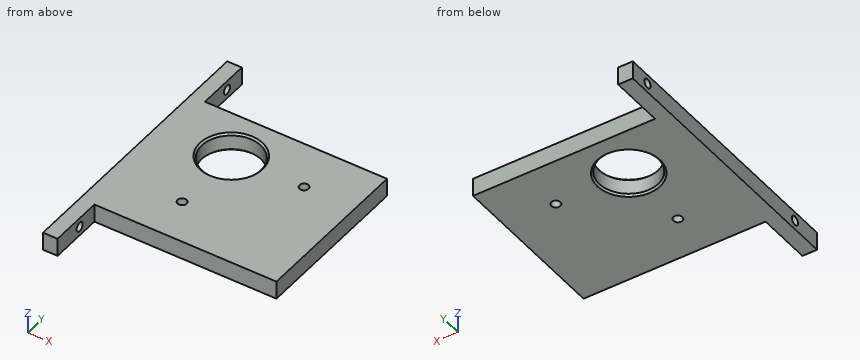
from build123d import *

# Parameters (mm, degrees)
SKETCH_1_R          = 8.1
EXTRUDE_1_DEPTH     = 5
SKETCH_2_R          = 1.25
CUT_EXTRUDE_1_DEPTH = 5
SKETCH_3_R          = 1.25
CUT_EXTRUDE_2_DEPTH = 120
CHAMFER_1_SIZE      = 0.5
SKETCH_4_W          = 16
SKETCH_4_H          = 45
CUT_EXTRUDE_3_DEPTH = 10


with BuildPart() as part:
    # 草图1 → 凸台-拉伸1 (new body)
    with BuildSketch(Plane.XY):
        Polygon((4, 60), (4, 75), (0, 75), (0, 0), (4, 0), (4, 15), (70, 15), (70, 60), align=None)
        with Locations((20, 47)):
            Circle(SKETCH_1_R, mode=Mode.SUBTRACT)
    extrude(amount=EXTRUDE_1_DEPTH)

    # 草图2 → 切除-拉伸1 (cut)
    with BuildSketch(Plane(origin=(4, 0, 0), x_dir=(0, 0, -1), z_dir=(1, 0, 0))):
        with Locations((-2.5, 69)):
            Circle(SKETCH_2_R)
        with Locations((-2.5, 9)):
            Circle(SKETCH_2_R)
    extrude(amount=-CUT_EXTRUDE_1_DEPTH, mode=Mode.SUBTRACT)

    # 草图3 → 切除-拉伸2 (cut)
    with BuildSketch(Plane(origin=(0, 0, 0), x_dir=(-1, 0, 0), z_dir=(0, 0, -1))):
        with Locations((-40, 47)):
            Circle(SKETCH_3_R)
        with Locations((-20, 27)):
            Circle(SKETCH_3_R)
    extrude(amount=-CUT_EXTRUDE_2_DEPTH, mode=Mode.SUBTRACT)

    # 倒角1
    chamfer_1_edges = [part.edges().sort_by_distance(p)[0] for p in [
        (11.9, 47, 0),
        (11.9, 47, 5),
    ]]
    chamfer(chamfer_1_edges, length=CHAMFER_1_SIZE)

    # 草图4 → 切除-拉伸3 (cut)
    with BuildSketch(Plane(origin=(0, 0, 0), x_dir=(-1, 0, 0), z_dir=(0, 0, -1))):
        with Locations((-62, 37.5)):
            Rectangle(SKETCH_4_W, SKETCH_4_H)
    extrude(amount=-CUT_EXTRUDE_3_DEPTH, mode=Mode.SUBTRACT)


solid = part.part
Build history of the part. All positions in model axes, mm. Coordinates: 2 decimals unless noted, no trailing zeros. Order: outer loops, then holes, each group sorted by start corner. A loop starts at its lowest first (then second) coordinate and runs counter-clockwise, first axis right, second up. Notation, with made-up numbers: (34.5, 82.25) - (90.5, 82.25) arc R29 ccw to (90.5, 116.25) - close; hole circle Ø7 at (89.5, 65.25). An arc over 180 degrees is marked (long way). Write each question's results on one line, items separated by ' | '. Start each with the question number.
Item 1: Band-saw the part on B-B on x = 40. Write the cut outline in (y, z).
Item 2: Wall check: probe 1 along Y at (x, z) = (0.9, 2.5); probe 2 along Y at (x, z) = (20, 1.7); probe 3 along X at (y, z) = (44, 4.35). Give the ranges that are in metal, low to high. Write a range as [from, to].
Item 3: Band-saw the part on C-C on y = 9. Write the cut outline in (x, z).
Item 4: Band-saw the part on A-A on z = 2.5. Write the cut outline in (x, y), and give its area (3 significant figures).
Item 5: Flat gauge pins, fed straight in: pin 1 (14.5 mm diameter, centred on x = 20, y = 47, fed in from +Z); pin 2 (2.5 mm diameter, centred on x = 41, z = 1.5, fed in from +Y); pin 3 (1.5 mm diameter, centred on y = 64, z = 3.5, fed in from +X); pin 4 (2.5 mm diameter, centred on x = 39, z = 2.5, fed in from -Y). Where does each tip first touch, or does it go through?
Numbers:
1) outline: (15, 0) - (45.75, 0) - (45.75, 5) - (15, 5) - close; (48.25, 0) - (60, 0) - (60, 5) - (48.25, 5) - close
2) probe 1: [0, 7.75], [10.25, 67.75], [70.25, 75] | probe 2: [15, 25.75], [28.25, 38.9], [55.1, 60] | probe 3: [0, 12.48], [27.52, 54]
3) outline: (0, 0) - (4, 0) - (4, 1.25) - (0, 1.25) - close; (0, 3.75) - (4, 3.75) - (4, 5) - (0, 5) - close
4) outline: (0, 0) - (4, 0) - (4, 7.75) - (0, 7.75) - close; (0, 10.25) - (4, 10.25) - (4, 15) - (54, 15) - (54, 60) - (4, 60) - (4, 67.75) - (0, 67.75) - close; (0, 70.25) - (4, 70.25) - (4, 75) - (0, 75) - close; hole circle Ø16.2 at (20, 47); hole circle Ø2.5 at (20, 27); hole circle Ø2.5 at (40, 47) | area: 2,310 mm^2
5) pin 1: through | pin 2: y = 60 | pin 3: x = 4 | pin 4: y = 15
